Geometry check sheet. Reference: the model listing, model coordinates, mm. A direction names the side the tool comes from. Give positions to 0.01 mm unless a question says otherwise; leave off trailing zeros. Write each loop counter-clockwise with the first axis right and the second up, starting at its lowest first coordinate (ties: lowest second). Pieces come first, ordered by that corner, then holes.
(1) Cross-section at A-A (y = 8). Record the boundary of the cut face in (x, z).
(2) Thickness scan on line 1 along Y through (x, z) = (0, -1.3); line 2 along X through (y, z) = (0, -0.9); line 3 along Y through (x, z) = (0, 0.2). Record the ranges inside material, lowest first.
(3) Cross-section at B-B (z = 0.55). Record the boundary of the cut face in (x, y).
(4) Cross-section at D-D (z = -1.15). Record the boundary of the cut face in (x, y).
(5) Cross-section at C-C (x = 0.5). Count the separate pieces of the cut face and the enclosed holes in it, and give its area (3 significant figures).
(6) Tool access check on faces 5 (the flat face through (-2, -8, 0)), 6 (the flat face through (2, -8, 0)), 7 (the cylindrical face through (-2.22, 4.83, -0.85)), 8 (the flat face through (2, 8, 0)), 9 (the cylindrical face through (0.03, 5.699, 0.285)). Record the directions out of +Z, -Z, +X, -X, +Y, -Y that give a thin tool (end or side, any length) a straight path to the whole face; none if there is none.
(7) Depth check by flat-ended pin: P1, Ø3, axis at x = -0.5, y = 3, coming from the +Z side; P2, Ø1.5, axis at y = -8.5, z = -1, coming from the +X side; P3, Ø1.5, axis at y = -8, z = -0.5, coming from the -X side. Enter the tip coordinate at first touch or a pass-through.
(8) Mould release check, pull along Y, two halves, no side actions. Record for faces 1 (the cylindrical face through (2.976, 0.937, -0.986)), 2 (the flat face through (3.3, 0.1, 0)), 3 (the flat face through (0, 7, 1)), 4 (the cylindrical face through (2.23, 4.81, -0.85)): +Y half, -Y half, draft (parallel to the pull), parting line (faces both ways), or undercut.
Autodesk Inventor part; units mm, degrees
ref_plane "YZ Plane" through (0, 0, 0) normal (1, 0, 0) x (0, 1, 0)
ref_plane "XZ Plane" through (0, 0, 0) normal (0, 1, 0) x (-1, 0, 0)
ref_plane "XY Plane" through (0, 0, 0) normal (0, 0, 1) x (1, 0, 0)
sketch "Sketch1" plane through (0, 0, 0) normal (0, 0, 1) x (1, 0, 0)
  circle A0 centre (0, 0) radius 3
  circle A1 centre (0, 0) radius 3
  circle A2 centre (0, 0) radius 5
  line L0 (0, 0) -> (0, 8)
  circle A3 centre (0, 8) radius 0.7
  line L1 (0, 0) -> (0, -8)
  circle A4 centre (0, -8) radius 0.7
  line L2 (-2, -10) -> (2, -10)
  line L3 (2, -10) -> (2, 10)
  line L4 (2, 10) -> (-2, 10)
  line L5 (-2, 10) -> (-2, -10)
  line L6 (-2, -10) -> (2, 10) construction
  line L7 (2, -10) -> (-2, 10) construction
  point P0 (-2, -4.5826)
  point P1 (2, -4.5826)
  point P2 (2, 4.5826)
  point P3 (-2, 4.5826)
  dimension "d0" = 6
  dimension "d1" = 10
  dimension "d2" = 8
  dimension "d3" = 1.4
  dimension "d4" = 8
  dimension "d5" = 1.4
  dimension "d6" = 4
  dimension "d7" = 20
extrude "Extrusion1" add sketch "Sketch1" against normal blind 2 contours A0 L3 A2 | A0 L0 A2 L3 | L3 A2 L1 A0 | A0 L5 A2 L0 | A2 L5 L4 L3 | L1 A2 L5 A0 | L3 L2 L5 A2 | A0 L5 A2
sketch "Sketch2" plane through (0, 0, 0) normal (0, 0, 1) x (1, 0, 0)
  arc A0 (-2, 4.5826) -> (-2, -4.5826) centre (0, 0) ccw
  line L0 (-2, -4.5826) -> (-2, -10)
  line L1 (-2, -10) -> (2, -10)
  line L2 (2, -10) -> (2, -4.5826)
  arc A1 (2, -4.5826) -> (2, 4.5826) centre (0, 0) ccw
  line L3 (2, 4.5826) -> (2, 10)
  line L4 (2, 10) -> (-2, 10)
  line L5 (-2, 10) -> (-2, 4.5826)
  circle A2 centre (0, -8) radius 0.7
  circle A3 centre (0, 8) radius 0.7
  circle A4 centre (0, 0) radius 3
  line L6 (-2, -10) -> (-2, -4.5826)
  line L7 (-2, -10) -> (-2, -6)
  line L8 (-2, -6) -> (2, -6)
  line L9 (2, -10) -> (2, -4.5826)
  line L10 (-2, 10) -> (-2, 4.5826)
  line L11 (-2, 10) -> (-2, 6)
  line L12 (-2, 6) -> (2, 6)
  line L13 (2, 10) -> (2, 4.5826)
  point P0 (2, 6)
  dimension "d10" = 4
  dimension "d11" = 4
extrude "Extrusion2" add sketch "Sketch2" along normal blind 1 contours L5 L4 L3 L12 | L8 L2 L1 L0
ref_plane "Work Plane1" through (0, -10, -2) normal (1, 0, 0) x (0, 0, -1)
chamfer "Chamfer1" distance 0.5 angle 45 4 edges at (-2, -10, -0.5) (2, -10, -0.5) (-2, 10, -0.5) (2, 10, -0.5)
fillet "Fillet1" radius 2 4 edges at (-2, -4.5826, -1) (-2, 4.5826, -1) (2, 4.5826, -1) (2, -4.5826, -1)
fillet "Fillet2" radius 1 2 edges at (0, -6, 0) (0, 6, 0)
thicken "Thicken1" operation add thickness 0.12 both sides no extend neighbours yes toward (0.9967573, -0.0804666, 0) faces at (2.9903, -0.2414, -1.3333)
properties part number "bearing_hh_1"
Reply:
1. outline: (-2, -2) - (-0.7, -2) - (-0.7, 1) - (-2, 1) - close; (0.7, -2) - (2, -2) - (2, 1) - (0.7, 1) - close
2. line 1: y = -10 to -8.7, -7.3 to -3.12, 3.12 to 7.3, 8.7 to 10
2. line 2: x = -5 to -3.12, 3.12 to 5
2. line 3: y = -10 to -8.7, -7.3 to -5.6, 5.6 to 7.3, 8.7 to 10
3. outline: (-2, -9.5) - (-1.5, -10) - (1.5, -10) - (2, -9.5) - (2, -5.89) - (-2, -5.89) - close; (-2, 5.89) - (2, 5.89) - (2, 9.5) - (1.5, 10) - (-1.5, 10) - (-2, 9.5) - close; hole circle Ø1.4 at (0, -8); hole circle Ø1.4 at (0, 8)
4. outline: (-2.86, -4.1) arc R2 cw to (-2, -5.74) - (-2, -9.5) - (-1.5, -10) - (1.5, -10) - (2, -9.5) - (2, -5.74) arc R2 cw to (2.86, -4.1) arc R5 ccw to (2.86, 4.1) arc R2 cw to (2, 5.74) - (2, 9.5) - (1.5, 10) - (-1.5, 10) - (-2, 9.5) - (-2, 5.74) arc R2 cw to (-2.86, 4.1) arc R5 ccw to start; hole circle Ø6.24 at (0, 0); hole circle Ø1.4 at (0, -8); hole circle Ø1.4 at (0, 8)
5. separate pieces: 4
5. enclosed holes: 0
5. area: 30.2 mm2
6. face 5: +Z, -Z, -X, -Y
6. face 6: +Z, -Z, +X, -Y
6. face 7: +Z, -Z, -X, +Y
6. face 8: +Z, -Z, +X, +Y
6. face 9: +Z, +X, -X
7. P1: stops at z = 0
7. P2: stops at x = 2
7. P3: stops at x = -2
8. face 1: undercut
8. face 2: undercut
8. face 3: draft
8. face 4: +Y half
